Can you work these out from the drawing? Everything is in mm from the part's minimum corner. Give positions to 0.01 mm unless a question says otherwise; leave off trailing zeros. Write each loop counter-clockwise with the first axis right and the second up, starting at its lowest first coordinate (ties: lowest second). Pieces come first, ordered by that corner, then holes. Notation, with made-up numbers: (79.25, 1.25) - (115.25, 1.25) arc R31 ccw to (115.25, 39.25) - close; hole circle Ø8 at (28.5, -26). An arc over 180 degrees is marked (long way). Return JSON: item names as keys, results as strings. Group by question number.
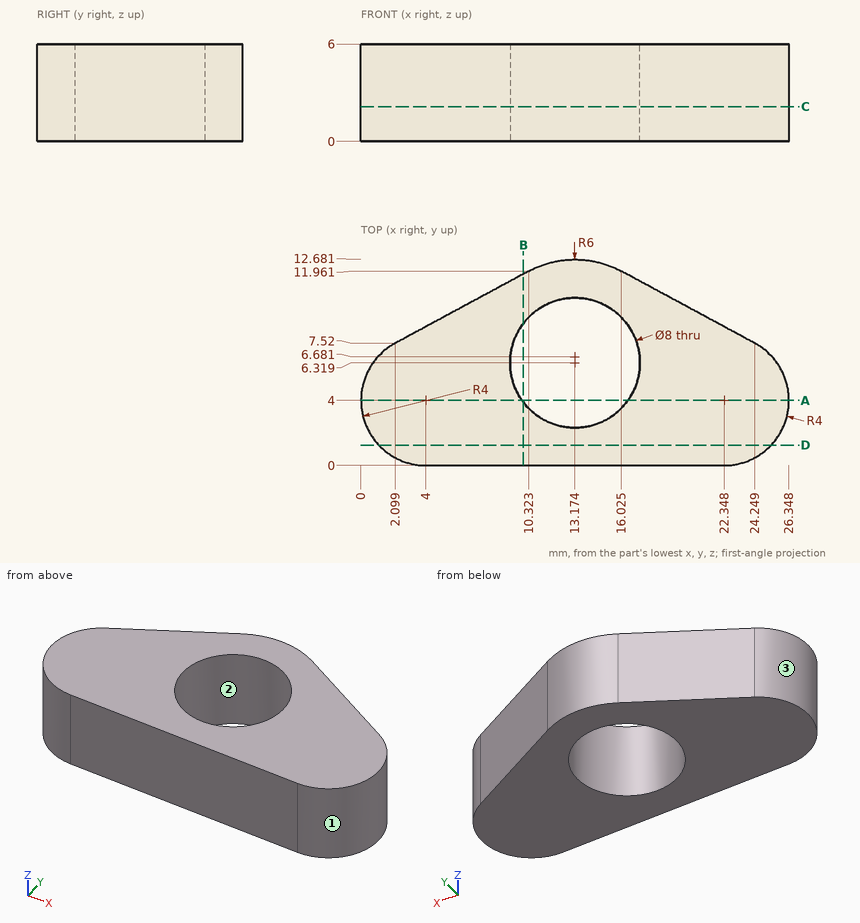
1) Imagine slicing it at C-C, the plane z = 2.15. Write out the boundary of the cut face in (x, y) (1 decimal), and give its area (3 significant figures).
2) Will these pins go through, and if not, where does the flat tip stop? pin 1 Ø1.5 at (y, z) = (6.5, 4) entering from -X; pin 2 Ø1 at (x, z) = (17.5, 1) entering from +Y (1 decimal); pin 3 Ø5 at (x, y) = (13.17, 6.32) entering from -Z; pin 4 Ø1 at (y, z) = (9.5, 2) entering from +X (1 decimal).
3) Imagine slicing it at D-D, the plane y = 1.25. Write out the boundary of the cut face in (x, z) (1 decimal), and give its area (3 significant figures).
4) Imagine slicing it at A-A, the plane y = 4. Write out the boundary of the cut face in (x, z) (1 decimal).
5) Imagine slicing it at B-B, the plane x = 10. Write out the boundary of the cut face in (y, z) (1 decimal), and give its area (3 significant figures).
6) We'd pull the mould along X, two halves only. Please class the marked faces 1, 2 and 3: pulls with the +X half, pulls with the -X half, needs draft (parallel to the pull), parting line crosses it, or undercut.
7) I need wall thicknesses on line 1 along X through (y, z) = (4.25, 0.65); line 2 along X through (y, z) = (6.25, 3.8) (1 decimal); line 3 along Y through (x, z) = (10.25, 1.85). Which ranges of each line are inside material? Lowest first, please.
Resolved:
{
 "1": {"outline": "(2.1, 7.5) arc R4 ccw to (4, 0) - (22.3, 0) arc R4 ccw to (24.2, 7.5) - (16, 12) arc R6 ccw to (10.3, 12) - close; hole circle Ø8 at (13.2, 6.3)", "area": "201 mm^2"},
 "2": {"pin 1": "x = 0.4", "pin 2": "y = 11.4", "pin 3": "through", "pin 4": "x = 21.5"},
 "3": {"outline": "(1.1, 0) - (25.3, 0) - (25.3, 6) - (1.1, 6) - close", "area": "145 mm^2"},
 "4": {"outline": "(0, 0) - (9.9, 0) - (9.9, 6) - (0, 6) - close; (16.4, 0) - (26.3, 0) - (26.3, 6) - (16.4, 6) - close"},
 "5": {"outline": "(0, 0) - (3.9, 0) - (3.9, 6) - (0, 6) - close; (8.8, 0) - (11.8, 0) - (11.8, 6) - (8.8, 6) - close", "area": "41.5 mm^2"},
 "6": {"face 1": "pulls with the +X half", "face 2": "undercut", "face 3": "pulls with the -X half"},
 "7": {"line 1": "0.01 to 9.75, 16.6 to 26.34", "line 2": "0.7 to 9.2, 17.2 to 25.7", "line 3": "0 to 3.59, 9.05 to 11.92"}
}
